Verification items for the finished model (mm, model axes). Face numbers are marked on the shaded views. A direction names the side the tool comes from. Coordinates: 2 decimals unless noted, no trailing zeros. Order: outer loops, then holes, each group sorted by start corner. A loop starts at its lowest first (then second) coordinate and runs counter-clockwise, first axis right, second up. Notation, with made-up numbers: M 70.5,-4 L 108.5,-4 A7 ccw 108.5,6 Z; hole C -31,83 d10. An arc over 180 degrees is marked long. Return JSON: item names as keys, results as strings. Group by question number.
Q1. Go/stop test with flat-tipped pins: pin 1 Ø5.5 at (x, z) = (24, -39.5) entering from +Y; pin 2 Ø2 at (x, z) = (-17.5, -40) entering from -Y; pin 3 Ø12 at (x, z) = (1.5, -30.5) entering from +Y; pin 4 Ø2.5 at (x, z) = (-21.5, 31) entering from +Y. Record where each tip stops, or that it passes through.
Q2. Section check A-A, the plane y = 8. Count the separate pieces of the cut face and the enclosed holes in it, then the cut area to 3 significant figures.
Q3. Section check D-D, the plane y = 40. Enter the section's corners in (x, z) (3 decimals).
Q4. Access from +Z, -Z, +X, -X, +Y, -Y to the whole of each face (thin tool, end or side, straight path). Record for the marked faces 4 and 5.
Q5. Mould release check, pull along X, two halves, no side actions. Record for the marked faces 1, 2 and 3: pulls with the +X half, pulls with the -X half, needs draft (parallel to the pull), parting line crosses it, or undercut.
Q6. Thickness scan on probe 1 along X at (y, z) = (6, 30) (3 decimals); probe 2 along X at (y, z) = (4, 30) (3 decimals); probe 3 along X at (y, z) = (55, 8.5) (3 decimals). Record the ranges inside material, lowest first.
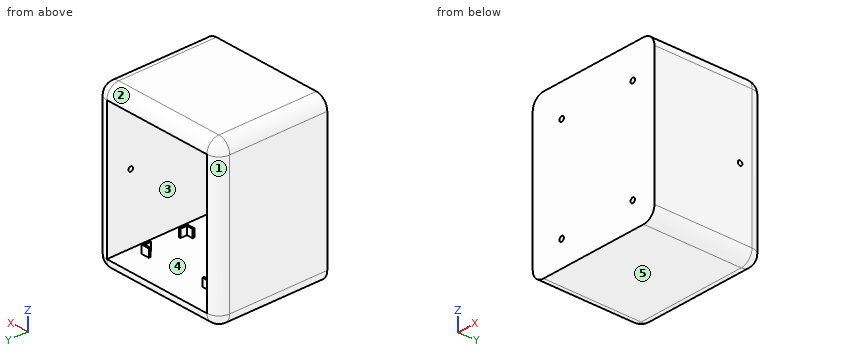
from build123d import *

# Parameters (mm, degrees)
SKETCH1_W               = 84.27
SKETCH1_H               = 100
BOSS_EXTRUDE1_DEPTH     = 68.8
SKETCH2_W               = 69.27
SKETCH2_H               = 85
CUT_EXTRUDE1_DEPTH      = 63.8
SKETCH6_W               = 5
SKETCH6_H               = 5
BOSS_EXTRUDE2_DEPTH     = 5
BOSS_EXTRUDE3_DEPTH     = 5
FILLET1_R               = 7.5
FILLET8_R               = 7.5
ADVANCEDHOLE2_OUTLINE_R = 1.5494
ADVANCEDHOLE2_DEPTH     = 10
HOLE1_START             = 34.635
HOLE1_OUTLINE_R         = 1.4224
HOLE1_DEPTH             = 7.5


# Read off the part's stored shape, not the designer's step: AdvancedHole2, Hole1
# Some blends are built 0.0001 mm under size
with BuildPart() as part:
    # Sketch1 → Boss-Extrude1 (new body)
    with BuildSketch(Plane(origin=(0, 0, 0), x_dir=(1, 0, 0), z_dir=(0, 1, 0))):
        Rectangle(SKETCH1_W, SKETCH1_H)
    extrude(amount=BOSS_EXTRUDE1_DEPTH)

    # Sketch2 → Cut-Extrude1 (cut)
    with BuildSketch(Plane(origin=(0, 68.8, 0), x_dir=(1, 0, 0), z_dir=(0, 1, 0))):
        Rectangle(SKETCH2_W, SKETCH2_H)
    extrude(amount=-CUT_EXTRUDE1_DEPTH, mode=Mode.SUBTRACT)

    # Sketch6 → Boss-Extrude2 (add)
    with BuildSketch(Plane(origin=(0, 5, 0), x_dir=(1, 0, 0), z_dir=(0, 1, 0))):
        with Locations((-22.135, 34.03)):
            Rectangle(SKETCH6_W, SKETCH6_H)
        with Locations((-22.135, -30)):
            Rectangle(SKETCH6_W, SKETCH6_H)
        with Locations((27.135, 34.03)):
            Rectangle(SKETCH6_W, SKETCH6_H)
        with Locations((27.135, -30)):
            Rectangle(SKETCH6_W, SKETCH6_H)
    extrude(amount=BOSS_EXTRUDE2_DEPTH)

    # Sketch7 → Boss-Extrude3 (add)
    with BuildSketch(Plane.XY.offset(-42.5)):
        Polygon((-19.635, 30), (-19.635, 25), (-14.635, 25), (-14.635, 26), (-18.635, 26), (-18.635, 30), align=None)
        Polygon((-19.635, 53.5), (-19.635, 48.5), (-18.635, 48.5), (-18.635, 52.5), (-14.635, 52.5), (-14.635, 53.5), align=None)
        Polygon((22.365, 53.5), (27.365, 53.5), (27.365, 48.5), (26.365, 48.5), (26.365, 52.5), (22.365, 52.5), align=None)
        Polygon((27.365, 30), (27.365, 25), (22.365, 25), (22.365, 26), (26.365, 26), (26.365, 30), align=None)
    extrude(amount=BOSS_EXTRUDE3_DEPTH)

    # Fillet1
    fillet1_edges = [part.edges().sort_by_distance(p)[0] for p in [
        (-42.135, 68.8, 0),
        (0, 68.8, 50),
        (42.135, 68.8, 0),
        (0, 68.8, -50),
    ]]
    fillet(fillet1_edges, radius=FILLET1_R - 0.0001)  # a hair under: the kernel refuses the full size

    # Fillet8
    # the kernel refuses this fillet: 7.5 mm, written as the material it takes off along each edge
    with BuildSketch(Plane(origin=(-34.635, 68.8, 42.5), x_dir=(-1, 0, 0), z_dir=(0, 0, -1))) as fillet8_piece_1:
        with BuildLine():
            CenterArc((0.0001, -7.4999), 7.4999, 0, 90)
            Line((7.5, -7.4999), (7.5, 0))
            Line((7.5, 0), (0.0001, 0))
        make_face()
    revolve(axis=Axis((-34.635, 68.8, 42.5), (0, 1, 0)), revolution_arc=90, mode=Mode.SUBTRACT)
    with BuildSketch(Plane(origin=(-34.635, 68.8, -42.5), x_dir=(0, 0, -1), z_dir=(1, 0, 0))) as fillet8_piece_2:
        with BuildLine():
            CenterArc((0.0001, -7.4999), 7.4999, 0, 90)
            Line((7.5, -7.4999), (7.5, 0))
            Line((7.5, 0), (0.0001, 0))
        make_face()
    revolve(axis=Axis((-34.635, 68.8, -42.5), (0, 1, 0)), revolution_arc=90, mode=Mode.SUBTRACT)
    with BuildSketch(Plane(origin=(34.635, 68.8, 42.5), x_dir=(0, 0, 1), z_dir=(-1, 0, 0))) as fillet8_piece_3:
        with BuildLine():
            CenterArc((0.0001, -7.4999), 7.4999, 0, 90)
            Line((7.5, -7.4999), (7.5, 0))
            Line((7.5, 0), (0.0001, 0))
        make_face()
    revolve(axis=Axis((34.635, 68.8, 42.5), (0, 1, 0)), revolution_arc=90, mode=Mode.SUBTRACT)
    with BuildSketch(Plane(origin=(34.635, 68.8, -42.5), x_dir=(1, 0, 0), z_dir=(0, 0, 1))) as fillet8_piece_4:
        with BuildLine():
            CenterArc((0.0001, -7.4999), 7.4999, 0, 90)
            Line((7.5, -7.4999), (7.5, 0))
            Line((7.5, 0), (0.0001, 0))
        make_face()
    revolve(axis=Axis((34.635, 68.8, -42.5), (0, 1, 0)), revolution_arc=90, mode=Mode.SUBTRACT)
    with BuildSketch(Plane(origin=(42.135, -18.75, -50), x_dir=(-1, 0, 0), z_dir=(0, 1, 0)), Plane(origin=(42.135, -18.75, 50), x_dir=(0, 0, -1), z_dir=(0, 1, 0))) as fillet8_piece_5:
        with BuildLine():
            CenterArc((FILLET8_R, FILLET8_R), FILLET8_R, 180, 90)
            Line((0, FILLET8_R), (0, 0))
            Line((0, 0), (FILLET8_R, 0))
        make_face()
    extrude(amount=87.55, mode=Mode.SUBTRACT)
    with BuildSketch(Plane(origin=(-42.135, -18.75, 50), x_dir=(0, 0, -1), z_dir=(0, 1, 0)), Plane(origin=(-42.135, -18.75, -50), x_dir=(1, 0, 0), z_dir=(0, 1, 0))) as fillet8_piece_6:
        with BuildLine():
            CenterArc((FILLET8_R, -FILLET8_R), FILLET8_R, 90, 90)
            Line((0, -FILLET8_R), (0, 0))
            Line((0, 0), (FILLET8_R, 0))
        make_face()
    extrude(amount=87.55, mode=Mode.SUBTRACT)

    # AdvancedHole2 outline → AdvancedHole2 (cut)
    with BuildSketch(Plane(origin=(0, 0, 0), x_dir=(1, 0, 0), z_dir=(0, 1, 0))):
        with Locations((-22.135, -30)):
            Circle(ADVANCEDHOLE2_OUTLINE_R)
        with Locations((27.135, -30)):
            Circle(ADVANCEDHOLE2_OUTLINE_R)
        with Locations((27.135, 34.03)):
            Circle(ADVANCEDHOLE2_OUTLINE_R)
        with Locations((-22.135, 34.03)):
            Circle(ADVANCEDHOLE2_OUTLINE_R)
    extrude(amount=ADVANCEDHOLE2_DEPTH, mode=Mode.SUBTRACT)

    # Hole1 outline → Hole1 (cut)
    with BuildSketch(Plane.YZ.offset(HOLE1_START)):
        with Locations((53.8, 0)):
            Circle(HOLE1_OUTLINE_R)
    extrude(amount=HOLE1_DEPTH, mode=Mode.SUBTRACT)


solid = part.part
Numbers:
{
 "1": {"pin 1": "stops at y = 53.5", "pin 2": "stops at y = 0", "pin 3": "stops at y = 5", "pin 4": "stops at y = 10"},
 "2": {"separate pieces": "5", "enclosed holes": "5", "area": "2,560 mm2"},
 "3": {"outline": "M -42.135,-42.5 A7.5 ccw -34.635,-50 L 34.635,-50 A7.5 ccw 42.135,-42.5 L 42.135,42.5 A7.5 ccw 34.635,50 L -34.635,50 A7.5 ccw -42.135,42.5 Z; hole M -34.635,-42.5 L 34.635,-42.5 L 34.635,42.5 L -34.635,42.5 Z"},
 "4": {"face 4": "none", "face 5": "-Z, +X, -X, +Y, -Y"},
 "5": {"face 1": "pulls with the -X half", "face 2": "needs draft", "face 3": "undercut"},
 "6": {"probe 1": "x = -42.135 to -34.635, -24.635 to -23.684, -20.586 to -19.635, 24.635 to 25.586, 28.684 to 29.635, 34.635 to 42.135", "probe 2": "x = -42.135 to -23.684, -20.586 to 25.586, 28.684 to 42.135", "probe 3": "x = -42.135 to -34.635, 34.635 to 42.135"}
}
